Autodesk Inventor part; units mm, degrees
ref_plane "YZ Plane" through (0, 0, 0) normal (1, 0, 0) x (0, 1, 0)
ref_plane "XZ Plane" through (0, 0, 0) normal (0, 1, 0) x (-1, 0, 0)
ref_plane "XY Plane" through (0, 0, 0) normal (0, 0, 1) x (1, 0, 0)
sketch "Sketch1" plane through (0, 0, 0) normal (0, 1, 0) x (-1, 0, 0)
  line L0 (50, -50) -> (-50, -50) construction
  line L1 (-50, -50) -> (-50, 50) construction
  line L2 (-50, 50) -> (50, 50) construction
  line L3 (50, 50) -> (50, -50) construction
  line L4 (54, -54) -> (-54, -54) construction
  line L5 (-54, -54) -> (-54, 54) construction
  line L6 (-54, 54) -> (54, 54) construction
  line L7 (54, 54) -> (54, -54) construction
  line L8 (58, -58) -> (-58, -58)
  line L9 (-58, -58) -> (-58, 58)
  line L10 (-58, 58) -> (58, 58)
  line L11 (58, 58) -> (58, -58)
  line L12 (54, -20) -> (50, -20)
  line L13 (50, -20) -> (50, 20)
  line L14 (50, 20) -> (54, 20)
  line L15 (54, 20) -> (54, -20)
  line L16 (-50, 20) -> (-54, 20)
  line L17 (-54, 20) -> (-54, -20)
  line L18 (-54, -20) -> (-50, -20)
  line L19 (-50, -20) -> (-50, 20)
  line L20 (-20, -50) -> (20, -50)
  line L21 (20, -50) -> (20, -54)
  line L22 (20, -54) -> (-20, -54)
  line L23 (-20, -54) -> (-20, -50)
  line L24 (20, 50) -> (-20, 50)
  line L25 (-20, 50) -> (-20, 54)
  line L26 (-20, 54) -> (20, 54)
  line L27 (20, 54) -> (20, 50)
  point P0 (0, 0)
  point P1 (0, -50)
  point P2 (50, 0)
  point P3 (50, 0)
  point P4 (0, -50)
  point P5 (52, 20)
  point P6 (52, -20)
  dimension "d0" = 4
  dimension "d1" = 4
  dimension "d2" = 100
  dimension "d3" = 100
  dimension "d4" = 40
extrude "Extrusion1" add sketch "Sketch1" along normal blind 4
properties part number "Top_100wx100d" material "Wood (Oak)"
Input: part model. Units: mm. Frame: model coordinates. A direction names the side the tool comes from. Round coordinates to 2 decimals unless told otherwise and drop trailing zeros. Loops run counter-clockwise (first coordinate to the right, second up) from the corner with the lowest first, then second, coordinate; pieces in that order, holes last. Notation, with made-up numbers: (59, -24) - (75, -24) arc R22 ccw to (75, 10) - close; hole circle Ø3 at (-32.5, 86.25). An arc over 180 degrees is marked (long way). One line per item, written item: value. Start each with the question number.
(1) Section C-C, the plane y = 0.7. Return loops of the section in (x, z).
(2) Ray query, line 1 (X direction, y = 0.2, z = 1); line 2 (Z direction, x = 52.5, y = 2.05). Return the intervals inside material, ascending. Write a range as [from, to].
(3) Draft query along Z for faces 3 (the flat face through (-58, 2, 1)), 4 (the flat face through (-54, 2, 0)). Return one class per face: +Z half, -Z half, draft (parallel to the pull), parting line (faces both ways), or undercut.
(4) Access query for faces 1 (the flat face through (-52, 2, -20)), 2 (the flat face through (1, 0, 1)). Directions: +Z, -Z, +X, -X, +Y, -Y. A direction counts if a zero-diameter tool reaches every point of the face in a straight line with its end or side. Return the directions, or none.
(5) Section B-B, the plane x = -13.5. Return loops of the section in (y, z), plus the area to 3 significant figures.
(6) Section A-A, the plane z = -6. Return loops of the section in (x, y), plus the area to 3 significant figures.
Results below:
1. outline: (-58, -58) - (58, -58) - (58, 58) - (-58, 58) - close; hole (-54, -20) - (-50, -20) - (-50, 20) - (-54, 20) - close; hole (-20, -54) - (20, -54) - (20, -50) - (-20, -50) - close; hole (-20, 50) - (20, 50) - (20, 54) - (-20, 54) - close; hole (50, -20) - (54, -20) - (54, 20) - (50, 20) - close
2. line 1: [-58, -54], [-50, 50], [54, 58]
2. line 2: [-58, -20], [20, 58]
3. face 3: draft
3. face 4: undercut
4. face 1: +Y, -Y
4. face 2: +Z, -Z, +X, -X, -Y
5. outline: (0, -58) - (4, -58) - (4, -54) - (0, -54) - close; (0, -50) - (4, -50) - (4, 50) - (0, 50) - close; (0, 54) - (4, 54) - (4, 58) - (0, 58) - close
5. area: 432 mm^2
6. outline: (-58, 0) - (-54, 0) - (-54, 4) - (-58, 4) - close; (-50, 0) - (50, 0) - (50, 4) - (-50, 4) - close; (54, 0) - (58, 0) - (58, 4) - (54, 4) - close
6. area: 432 mm^2
